from build123d import *

# Parameters (mm, degrees)
F0_R     = 2.5
F1_DEPTH = 2.29


with BuildPart() as f1:
    # F0 (on Top) → F1 (new body, symmetric)
    with BuildSketch(Plane.XY):
        with BuildLine():
            Line((3.4641016151, -2), (3.4641016151, 0))
            Line((3.4641016151, 0), (3.4641016151, 2))
            ThreePointArc((3.4641016151, 2), (-4, 0), (3.4641016151, -2))
        make_face()
        Circle(F0_R, mode=Mode.SUBTRACT)
        with BuildLine():
            Line((4, 0), (3.4641016151, 0))
            Line((3.4641016151, 0), (3.4641016151, -2))
            ThreePointArc((3.4641016151, -2), (3.8637033052, -1.0352761804), (4, 0))
        make_face()
        with BuildLine():
            Line((3.4641016151, 2), (3.4641016151, 0))
            Line((3.4641016151, 0), (4, 0))
            ThreePointArc((4, 0), (3.8637033052, 1.0352761804), (3.4641016151, 2))
        make_face()
        with BuildLine():
            Line((13.4641016151, 0), (4, 0))
            ThreePointArc((4, 0), (3.8637033052, -1.0352761804), (3.4641016151, -2))
            Line((3.4641016151, -2), (13.4641016151, -2))
            Line((13.4641016151, -2), (13.4641016151, 0))
        make_face()
        with BuildLine():
            ThreePointArc((3.4641016151, 2), (3.8637033052, 1.0352761804), (4, 0))
            Line((4, 0), (13.4641016151, 0))
            Line((13.4641016151, 0), (13.4641016151, 2))
            Line((13.4641016151, 2), (3.4641016151, 2))
        make_face()
        Polygon((14.4215287229, 0), (13.4641016151, 0), (13.4641016151, -2), align=None)
        Polygon((13.4641016151, 2), (13.4641016151, 0), (14.4215287229, 0), align=None)
        Polygon((16.3363829384, 0), (14.4215287229, 0), (14.9002422768, -1), align=None)
        Polygon((14.9002422768, 1), (14.4215287229, 0), (16.3363829384, 0), align=None)
        Polygon((14.4215287229, 0), (13.4641016151, -2), (14.9002422768, -1), align=None)
        with BuildLine():
            Line((14.9002422768, -1), (13.4641016151, -2))
            ThreePointArc((13.4641016151, -2), (15.841018376, -4.7031302683), (19.3898786666, -5.3049916919))
            Line((19.3898786666, -5.3049916919), (18.4641016151, -3.7014988023))
            ThreePointArc((18.4641016151, -3.7014988023), (16.2280789653, -2.9497959409), (14.9002422768, -1))
        make_face()
        Polygon((16.3363829384, 0), (14.9002422768, -1), (52.2525225805, -1), (55, 0), align=None)
        Polygon((52.2525225805, 1), (14.9002422768, 1), (16.3363829384, 0), (55, 0), align=None)
        with BuildLine():
            ThreePointArc((19.3898786666, 5.3049916919), (15.841018376, 4.7031302683), (13.4641016151, 2))
            Line((13.4641016151, 2), (14.9002422768, 1))
            ThreePointArc((14.9002422768, 1), (16.2280789653, 2.9497959409), (18.4641016151, 3.7014988023))
            Line((18.4641016151, 3.7014988023), (19.3898786666, 5.3049916919))
        make_face()
        Polygon((14.9002422768, 1), (13.4641016151, 2), (14.4215287229, 0), align=None)
    extrude(amount=F1_DEPTH, both=True)


solid = f1.part
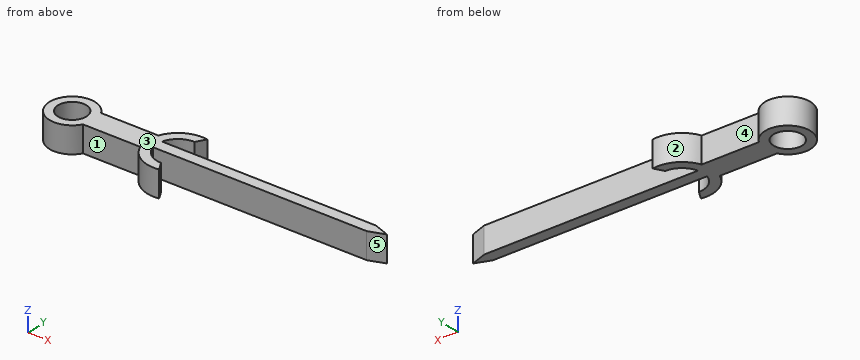
Verification items for the finished model (mm, model axes). Face numbers are marked on the shaded views. A direction names the side the tool comes from. Coordinates: 2 decimals unless noted, no trailing zeros. Loops run counter-clockwise (first coordinate to the right, second up) from the corner with the lowest first, then second, coordinate; pieces in that order, holes last. Notation, with made-up numbers: (-27.5, -18) -> (3.5, -18) arc R21 cw to (3.5, 10) -> close; hole circle Ø2 at (27, 30.5). An arc over 180 degrees is marked (long way). Write each question's results on one line, items separated by ' | '.
Item 1: Mould release check, pull along X, two halves, no side actions. Record for the marked faces 3, 4 and 5: +X half, -X half, draft (parallel to the pull), parting line (faces both ways), or undercut.
Found:
face 3: draft | face 4: undercut | face 5: +X half
Item 2: Section check C-C, the plane y = 3. Enter the section's corners in (x, z), plus the area to 3 significant figures.
Found:
outline: (-2.65, -2.29) -> (2.65, -2.29) -> (2.65, 2.29) -> (-2.65, 2.29) -> close; (13.99, -2.29) -> (16.3, -2.29) -> (16.3, 2.29) -> (13.99, 2.29) -> close | area: 34.8 mm2
Item 3: Section check D-D, the plane x = 38. Enter the section's corners in (y, z), plus the area to 3 significant figures.
Found:
outline: (-1, -2.29) -> (1, -2.29) -> (1, 2.29) -> (-1, 2.29) -> close | area: 9.16 mm2
Item 4: Gauge pin test, flat ends, axial feed: pin 1 (1 mm diameter, centred on x = 13, z = -0.5, fed in from +Y); pin 2 (1.5 mm diameter, centred on x = 13.5, z = 2, fed in from +Y); pin 3 (2.5 mm diameter, centred on x = 34, z = 1, fed in from +Y). Record the tip position at first contact, or that the pin passes through.
Found:
pin 1: stops at y = 2.09 | pin 2: stops at y = 3.35 | pin 3: stops at y = 1
Item 5: Material ranges on L1, parallel to Y at x = 0, z = 1; L2, parallel to Y at x = 49, z = 1.6; L3, parallel to X at y = 2.25, z = 1.7, recorded low to high.
Found:
L1: y = -4 to -2.5, 2.5 to 4 | L2: y = -1 to 1 | L3: x = -3.31 to -1.09, 1.09 to 3.31, 13.57 to 15.52
Item 6: Section check B-B, the plane x = 0. Enter the section's corners in (y, z), plus the area to 3 significant figures.
Found:
outline: (-4, -2.29) -> (-2.5, -2.29) -> (-2.5, 2.29) -> (-4, 2.29) -> close; (2.5, -2.29) -> (4, -2.29) -> (4, 2.29) -> (2.5, 2.29) -> close | area: 13.7 mm2
Item 7: Section check A-A, the plane z = -1. Enter the section's corners in (x, y) (1 decimal).
Found:
outline: (3.5, -2) -> (13.5, -2) arc R5.4 ccw to (19.4, -5.3) -> (18.5, -3.7) arc R3.7 cw to (14.9, -1) -> (52.3, -1) -> (55, 0) -> (52.3, 1) -> (14.9, 1) arc R3.7 cw to (18.5, 3.7) -> (19.4, 5.3) arc R5.4 ccw to (13.5, 2) -> (3.5, 2) arc R4 ccw (long way) to start; hole circle Ø5 at (0, 0)
Item 8: Tool access check on the marked faces 1 and 2. Record the directions out of +Z, -Z, +X, -X, +Y, -Y that give a thin tool (end or side, any length) a straight path to the whole face; none if there is none.
Found:
face 1: +Z, -Z, -Y | face 2: +Z, -Z, +Y
